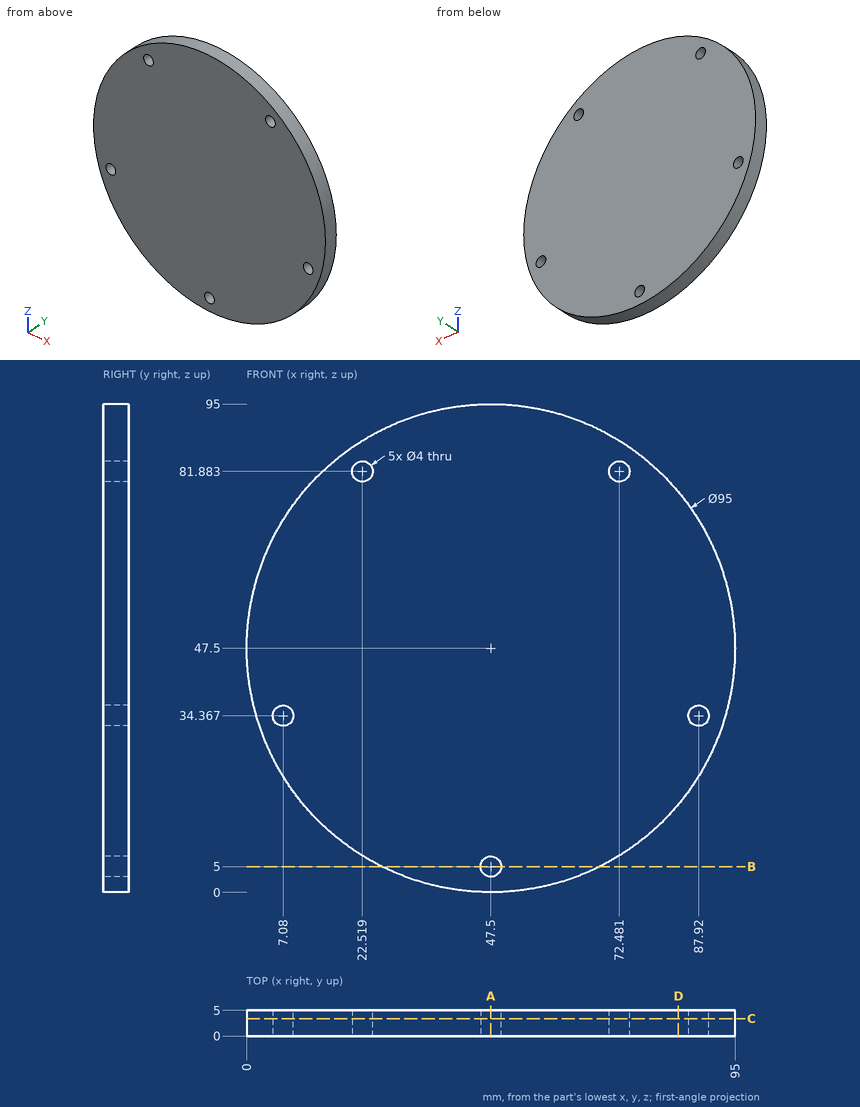
Design review of the part shown in the three views and the two pictorial views. Dimensions are in mm from the part's minimum x, y and z. Round coordinates to 2 decimals unless told otherwise and drop trailing zeros. Order: outer loops, then holes, each group sorted by start corner. A loop starts at its lowest first (then second) coordinate and runs counter-clockwise, first axis right, second up. Notation, with made-up numbers: (19, 85) - (45, 85) arc R23 cw to (45, 98) - close; hole circle Ø5 at (42, 9.5). An arc over 180 degrees is marked (long way). Answer in a Markdown table with one row per item.
(1) Take a section at D-D on x = 84. Write out the cut boundary in (y, z).
Result set:
| item | result |
|---|---|
| outline | (0, 17.1) - (5, 17.1) - (5, 77.9) - (0, 77.9) - close |
(2) Take a section at C-C on y = 3.4. Write out the cut boundary in (x, z), plus the area to 3 significant figures.
Result set:
| item | result |
|---|---|
| outline | circle Ø95 at (47.5, 47.5); hole circle Ø4 at (7.08, 34.37); hole circle Ø4 at (22.52, 81.88); hole circle Ø4 at (47.5, 5); hole circle Ø4 at (72.48, 81.88); hole circle Ø4 at (87.92, 34.37) |
| area | 7,030 mm2 |
(3) Take a section at B-B on z = 5. Write out the cut boundary in (x, y).
Result set:
| item | result |
|---|---|
| outline | (26.29, 0) - (45.5, 0) - (45.5, 5) - (26.29, 5) - close; (49.5, 0) - (68.71, 0) - (68.71, 5) - (49.5, 5) - close |
(4) For line 1 (X direction, y = 3, z = 81.5) (1 decimal); line 2 (Z direction, x = 47.5, y = 1); line 3 (X direction, y = 0.45, z = 80.5) (1 decimal), list the stretches that pass through material, from the lowest coordinate up. Write a range as from..to.
Result set:
| item | result |
|---|---|
| line 1 | x = 14.3..20.6, 24.5..70.5, 74.4..80.7 |
| line 2 | z = 0..3, 7..95 |
| line 3 | x = 13.3..21.1, 24..71, 73.9..81.7 |
(5) Clearance check with a flat-ended pin moving along its axis: P1, Ø1, axis at y = 0.5, z = 41, coming from the +X side. State where the tip first meets the part, or that it passes through.
Result set:
| item | result |
|---|---|
| P1 | stops at x = 94.62 |
(6) Take a section at A-A on x = 47.5. Write out the cut boundary in (y, z), plus the area to 3 significant figures.
Result set:
| item | result |
|---|---|
| outline | (0, 0) - (5, 0) - (5, 3) - (0, 3) - close; (0, 7) - (5, 7) - (5, 95) - (0, 95) - close |
| area | 455 mm2 |
